```python
from build123d import *

# Parameters (mm, degrees)
F1_DEPTH = 6.35
F0_R     = 21.5364
F2_DEPTH = 25.4
F3_W     = 27.747467
F3_H     = 9.982902
F4_DEPTH = 18.9484
F6_DEPTH = 25.4


with BuildPart() as f1:
    # F0 (on Top) → F1 (new body)
    with BuildSketch(Plane.XY):
        with BuildLine():
            ThreePointArc((-11.211676, -28.56255), (-30.684213, 0), (-11.211676, 28.56255))
            Line((-11.211676, 28.56255), (-62.113033, 28.56255))
            Line((-62.113033, 28.56255), (-62.113033, -28.56255))
            Line((-62.113033, -28.56255), (-11.211676, -28.56255))
        make_face()
    extrude(amount=F1_DEPTH)

    # F0 (on Top) → F2 (join)
    with BuildSketch(Plane.XY):
        with BuildLine():
            ThreePointArc((-11.211676, -28.56255), (17.284379, -25.352933), (30.684213, 0))
            ThreePointArc((30.684213, 0), (17.284379, 25.352933), (-11.211676, 28.56255))
            ThreePointArc((-11.211676, 28.56255), (-30.684213, 0), (-11.211676, -28.56255))
        make_face()
        Circle(F0_R, mode=Mode.SUBTRACT)
    extrude(amount=F2_DEPTH)

    # F3 (on face) → F4 (join)
    with BuildSketch(Plane.XY.offset(6.35)):
        with Locations((-44.115293, 0.20172)):
            Rectangle(F3_W, F3_H)
    extrude(amount=F4_DEPTH)

    # F5 (on face) → F6 (cut)
    with BuildSketch(Plane.XZ.offset(4.789731)):
        Polygon((-57.989027, 6.35), (-30.308075, 25.2984), (-57.989027, 25.2984), align=None)
    extrude(amount=-F6_DEPTH, mode=Mode.SUBTRACT)


solid = f1.part
```
For this review, take the finished solid that the model builds, in its own axes (mm). A direction names the side the tool comes from. Round coordinates to 2 decimals unless told otherwise and drop trailing zeros. Loops run counter-clockwise (first coordinate to the right, second up) from the corner with the lowest first, then second, coordinate; pieces in that order, holes last.
(1) We need section A-A (x = 0). Give the boundary of the cut face in (y, z).
Returned:
outline: (-30.68, 0) - (-21.54, 0) - (-21.54, 25.4) - (-30.68, 25.4) - close; (21.54, 0) - (30.68, 0) - (30.68, 25.4) - (21.54, 25.4) - close
(2) Tool access review of faces 4 (the flat face through (-43, 7, 6.35)), 5 (the flat face through (-27, 0, 0)), 6 (the flat face through (-41, 5.193, 14)), 7 (the flat face through (-36, 28.563, 3)), 8 (the flat face through (-37, -28.563, 3)): name each direction out of +Z, -Z, +X, -X, +Y, -Y from which nothing blocks a thin tool from reaching the whole face with its end or side.
Returned:
face 4: +Z, -X
face 5: -Z, +X, -X, +Y, -Y
face 6: +Z, -X, +Y
face 7: +Z, -Z, -X, +Y
face 8: +Z, -Z, -X, -Y
(3) Mouldability with a two-part tool opening along Y and no side actions: class faces 1 (the cylindrical face through (20.54, 6.47, 12.52)), 2 (the flat face through (-21, -6, 25.4)), 3 (the flat face through (-41, -4.79, 11)) as released by +Y, released by -Y, zero draft, split by the parting line, or undercut.
Returned:
face 1: undercut
face 2: zero draft
face 3: released by -Y
(4) Clearance check with flat-ended pins moving along their axes: P1, Ø15, axis at x = -47.5, z = 17.5, coming from the +Y side; P2, Ø3, axis at x = 10.5, z = 16.5, coming from the -Y side; P3, Ø12, axis at x = -25.5, z = 22.5, coming from the -Y side; P4, Ø6, axis at y = -2, z = 20.5, coming from the +X side. State where each tip first meets the part, or that it passes through.
Returned:
P1: stops at y = 5.19
P2: stops at y = -29.33
P3: stops at y = -23.69
P4: stops at x = 30.68
(5) We need section C-C (y = 16.5). Give the boundary of the cut face in (x, z), plus the area to 3 significant figures.
Returned:
outline: (-62.11, 0) - (-13.84, 0) - (-13.84, 25.4) - (-25.87, 25.4) - (-25.87, 6.35) - (-62.11, 6.35) - close; (13.84, 0) - (25.87, 0) - (25.87, 25.4) - (13.84, 25.4) - close
area: 841 mm2
(6) Wall thickness on line 1 along Y through (x, z) = (0, 11.75); line 2 along Y through (x, z) = (-1.5, 6.5); line 3 along Z through (x, y) = (-37.5, 20.5): over which ranges is each line inside the solid? List them lowest first.
Returned:
line 1: y = -30.68 to -21.54, 21.54 to 30.68
line 2: y = -30.65 to -21.48, 21.48 to 30.65
line 3: z = 0 to 6.35
(7) We need section D-D (x = -51.5). Give the boundary of the cut face in (y, z).
Returned:
outline: (-28.56, 0) - (28.56, 0) - (28.56, 6.35) - (5.19, 6.35) - (5.19, 10.79) - (-4.79, 10.79) - (-4.79, 6.35) - (-28.56, 6.35) - close
(8) We need section B-B (z = 4). Give the boundary of the cut face in (x, y).
Returned:
outline: (-62.11, -28.56) - (-11.21, -28.56) arc R30.68 ccw to (30.68, 0) arc R30.68 ccw to (-11.21, 28.56) - (-62.11, 28.56) - close; hole circle Ø43.07 at (0, 0)
